Answer from the drawing. Dimensions are ordinates in mm from the lowest x, y and z of the part. A direction names the side the tool comes from. Coordinates: 2 decimals unless noted, no trailing zeros. Write each loop counter-clockwise with the first axis right and the second up, starting at its lowest first coordinate (ties: lowest second). Pieces come first, ordered by that corner, then holes. Notation, with made-up numbers: (-40, -3.5) - (-23, -3.5) arc R4 ccw to (-23, 0.5) - close; hole circle Ø6 at (89.5, 58.25). An arc over 180 degrees is marked (long way). Use a Markdown table: item, result.
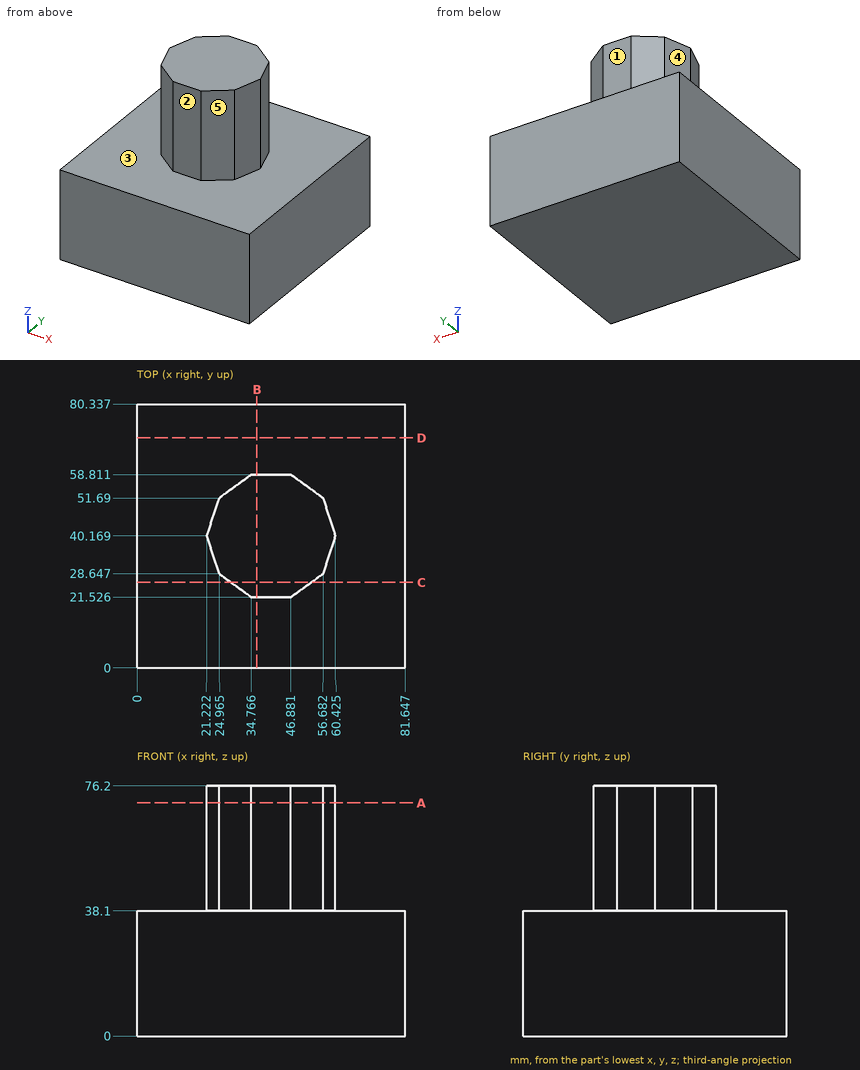
(1) A cutting plane is placed at D-D, the plane y = 70. Write down the section's boundary in (x, z).
Report:
| item | result |
|---|---|
| outline | (0, 0) - (81.65, 0) - (81.65, 38.1) - (0, 38.1) - close |
(2) A cutting plane is placed at B-B, the plane x = 36.5. Write down the section's boundary in (y, z), and give its area (3 significant figures).
Report:
| item | result |
|---|---|
| outline | (0, 0) - (80.34, 0) - (80.34, 38.1) - (58.81, 38.1) - (58.81, 76.2) - (21.53, 76.2) - (21.53, 38.1) - (0, 38.1) - close |
| area | 4,480 mm² |
(3) A cutting plane is placed at C-C, the plane y = 26. Write down the section's boundary in (x, z), and give its area (3 significant figures).
Report:
| item | result |
|---|---|
| outline | (0, 0) - (81.65, 0) - (81.65, 38.1) - (53.04, 38.1) - (53.04, 76.2) - (28.61, 76.2) - (28.61, 38.1) - (0, 38.1) - close |
| area | 4,040 mm² |
(4) For the marked faces 1, 2, 3, 4 and 5, determine the directions among +Z, -Z, +X, -X, +Y, -Y from which every point of the face is accessible in a straight line to the end or side of a thin tool.
Report:
| item | result |
|---|---|
| face 1 | +Z, +X, -X, +Y |
| face 2 | +Z, +X, -X, -Y |
| face 3 | +Z |
| face 4 | +Z, -X, +Y |
| face 5 | +Z, +X, -Y |
(5) Straight lines are drawn through the part: L1, parallel to Z at x = 66.5, y = 15.5; L2, parallel to Y at x = 53.5, z = 50 (1 decimal); L3, parallel to X at y = 42, z = 72. For each, find the intervals that lie inside material, in ascending order.
Report:
| item | result |
|---|---|
| L1 | z = 0 to 38.1 |
| L2 | y = 26.3 to 54 |
| L3 | x = 21.82 to 59.83 |
(6) A cutting plane is placed at A-A, the plane z = 71. Write down the section's boundary in (x, y) (1 decimal), and give its area (3 significant figures).
Report:
| item | result |
|---|---|
| outline | (21.2, 40.2) - (25, 28.6) - (34.8, 21.5) - (46.9, 21.5) - (56.7, 28.6) - (60.4, 40.2) - (56.7, 51.7) - (46.9, 58.8) - (34.8, 58.8) - (25, 51.7) - close |
| area | 1,130 mm² |
(7) Each of these flat-tipped pins is pushed along its axis until it touches: P1, Ø2, axis at x = 26, y = 24.5, coming from the +Z side; P2, Ø3.5, axis at x = 41, z = 53.5, coming from the -Y side; P3, Ø3.5, axis at x = 38, z = 61.5, coming from the +Y side. Where does it stop, or does it pass through?
Report:
| item | result |
|---|---|
| P1 | stops at z = 38.1 |
| P2 | stops at y = 21.53 |
| P3 | stops at y = 58.81 |
